Autodesk Inventor part; units mm, degrees
ref_plane "YZ Plane" through (0, 0, 0) normal (1, 0, 0) x (0, 1, 0)
ref_plane "XZ Plane" through (0, 0, 0) normal (0, 1, 0) x (-1, 0, 0)
ref_plane "XY Plane" through (0, 0, 0) normal (0, 0, 1) x (1, 0, 0)
sketch "Sketch1" plane through (0, 0, 0) normal (0, 0, 1) x (1, 0, 0)
  line L0 (-25.4, 38.1) -> (25.4, 38.1)
  line L1 (25.4, 38.1) -> (25.4, -38.1)
  line L2 (25.4, -38.1) -> (-25.4, -38.1)
  line L3 (-25.4, -38.1) -> (-25.4, 38.1)
  circle A0 centre (0, 0) radius 21.59
  circle A1 centre (-20.32, 33.02) radius 2.286
  circle A2 centre (0, 0) radius 19.05 construction
  circle A3 centre (20.32, 33.02) radius 2.286
  circle A4 centre (-20.32, -33.02) radius 2.286
  circle A5 centre (20.32, -33.02) radius 2.286
  point P0 (-17.145, 19.05)
  point P1 (17.145, 19.05)
  point P2 (17.145, -19.05)
  point P3 (-17.145, -19.05)
  dimension "d0" = 43.18
  dimension "d1" = 76.2
  dimension "d2" = 38.1
  dimension "d3" = 50.8
  dimension "d4" = 25.4
  dimension "d5" = 4.572
  dimension "d6" = 5.08
  dimension "d7" = 5.08
  dimension "d8" = 38.1
  dimension "d9" = 4.572
  dimension "d10" = 5.08
  dimension "d11" = 5.08
  dimension "d12" = 4.572
  dimension "d13" = 4.572
  dimension "d20" = 66.04
  dimension "d21" = 40.64
  dimension "d23" = 34.29
  dimension "d24" = 19.05
  dimension "d25" = 19.05
  dimension "d26" = 17.145
extrude "Extrusion1" add sketch "Sketch1" against normal blind 3.175
sketch "Sketch2" plane through (0, 0, -3.175) normal (0, 0, -1) x (-1, 0, 0)
  circle A0 centre (-20.32, -33.02) radius 2.286
  circle A1 centre (20.32, -33.02) radius 2.286
  circle A2 centre (-20.32, 33.02) radius 2.286
  circle A3 centre (20.32, 33.02) radius 2.286
  line L0 (25.4, 38.1) -> (25.4, -38.1)
  line L1 (-25.4, 38.1) -> (25.4, 38.1)
  line L2 (-25.4, -38.1) -> (-25.4, 38.1)
  line L3 (25.4, -38.1) -> (-25.4, -38.1)
  line L4 (-25.4, 38.1) -> (25.4, 38.1)
  line L5 (25.4, 38.1) -> (25.4, 29.845)
  line L6 (25.4, 29.845) -> (-25.4, 29.845)
  line L7 (-25.4, 29.845) -> (-25.4, 38.1)
  line L8 (-25.4, -38.1) -> (25.4, -38.1)
  line L9 (25.4, -38.1) -> (25.4, -29.845)
  line L10 (25.4, -29.845) -> (-25.4, -29.845)
  line L11 (-25.4, -29.845) -> (-25.4, -38.1)
  dimension "d16" = 8.255
  dimension "d17" = 8.255
extrude "Extrusion2" add sketch "Sketch2" along normal blind 5.08 contours L0 L6 L2 L1 | L0 L3 L2 L10
hole "Hole1" at (-17.145, 19.05, 0) at (17.145, 19.05, 0) at (17.145, -19.05, 0) at (-17.145, -19.05, 0) direction (0, 0, -1) diameter 3.302 end through all
equation "\"d9\" = d5"
equation "\"d12\" = d5"
equation "\"d13\" = d5"
equation "\"d17\" = d16"
properties part number "Dewalt CAP Clamp Plate"
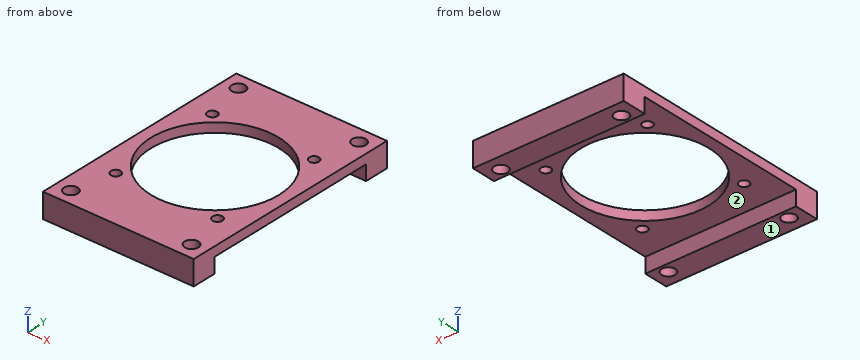
Source: CAD feature listing. Evaluate the final solid. Frame: model axes, mm. Face numbers are marked on the shaded views. A direction names the side the tool comes from. Give positions to 0.01 mm unless a question says otherwise; leave off trailing zeros. Write each loop counter-clockwise with the first axis right and the second up, starting at its lowest first coordinate (ties: lowest second). Pieces come first, ordered by that corner, then holes. Notation, with made-up numbers: M -17,-13.75 L 24,-13.75 A29 ccw 24,22.25 Z; hole C 70,57 d4. An arc over 180 degrees is marked long. Answer as a JSON object with one key per item and string values.
Q1. Ray query, line 1 along X through (y, z) = (-33.02, -3.75); line 2 along Y through (x, z) = (3, -3.75) (3 decimals); line 3 along X through (y, z) = (19.05, -1.65). Return the intervals inside material, ascending.
Geometry check:
{"line 1": "x = -25.4 to -22.61, -18.03 to 18.03, 22.61 to 25.4", "line 2": "y = -38.1 to -29.845, 29.845 to 38.1", "line 3": "x = -25.4 to -18.8, -15.49 to -10.16, 10.16 to 15.49, 18.8 to 25.4"}
Q2. Contact query for flat-ended pins moving along their axis: P1, Ø3, axis at x = 17.145, y = 19.05, coming from the -Z side; P2, Ø8, axis at x = 3.5, y = 22.5, coming from the -Z side (3 decimals). Output: stop coordinate, or through.
Geometry check:
{"P1": "passes through", "P2": "stops at z = -3.175"}
Q3. Access query for the marked faces 1 and 2. Directions: +Z, -Z, +X, -X, +Y, -Y. A direction counts if a zero-diameter tool reaches every point of the face in a straight line with its end or side. Return the directions, or none.
Geometry check:
{"face 1": "-Z, +X, -X, +Y, -Y", "face 2": "-Z, +X, -X"}
Q4. Cut plane A-A, the plane z = -4. Return the cut outline in (x, y) (3 decimals), then the cut area to 3 significant figures.
Geometry check:
{"outline": "M -25.4,-38.1 L 25.4,-38.1 L 25.4,-29.845 L -25.4,-29.845 Z; M -25.4,29.845 L 25.4,29.845 L 25.4,38.1 L -25.4,38.1 Z; hole C -20.32,-33.02 d4.572; hole C -20.32,33.02 d4.572; hole C 20.32,-33.02 d4.572; hole C 20.32,33.02 d4.572", "area": "773 mm^2"}
Q5. Cut plane B-B, the plane y = -33.02. Return the cut outline in (x, z) (3 decimals), then the cut area to 3 significant figures.
Geometry check:
{"outline": "M -25.4,-8.255 L -22.606,-8.255 L -22.606,0 L -25.4,0 Z; M -18.034,-8.255 L 18.034,-8.255 L 18.034,0 L -18.034,0 Z; M 22.606,-8.255 L 25.4,-8.255 L 25.4,0 L 22.606,0 Z", "area": "344 mm^2"}
Q6. Cut plane D-D, the plane y = -19.05. Return the cut outline in (x, z) (3 decimals), then the cut area to 3 significant figures.
Geometry check:
{"outline": "M -25.4,-3.175 L -18.796,-3.175 L -18.796,0 L -25.4,0 Z; M -15.494,-3.175 L -10.16,-3.175 L -10.16,0 L -15.494,0 Z; M 10.16,-3.175 L 15.494,-3.175 L 15.494,0 L 10.16,0 Z; M 18.796,-3.175 L 25.4,-3.175 L 25.4,0 L 18.796,0 Z", "area": "75.8 mm^2"}
Q7. Cut plane C-C, the plane x = 0. Return the cut outline in (y, z) (3 decimals), then the cut area to 3 significant figures.
Geometry check:
{"outline": "M -38.1,-8.255 L -29.845,-8.255 L -29.845,-3.175 L -21.59,-3.175 L -21.59,0 L -38.1,0 Z; M 21.59,-3.175 L 29.845,-3.175 L 29.845,-8.255 L 38.1,-8.255 L 38.1,0 L 21.59,0 Z", "area": "189 mm^2"}
